Here's the drawing with two shaded views (mm, measured from the low corner). I have some questions. A direction names the side the tool comes from. Coordinates: 2 decimals unless noted, no trailing zeros. Write each loop counter-clockwise with the first axis right and the second up, starting at its lowest first coordinate (ties: lowest second). Pieces come first, ordered by that corner, then holes.
Item 1: If I drill on probe 1 along X at (y, z) = (16, 4.75); probe 2 along Y at (x, z) = (37, 3.05); probe 3 along Y at (x, z) = (15, 3.75), over which ranges is the centre line in solid material (lowest first)?
Item 2: Thinking about a two-plate mould opening in X: for the marked faces 5, 6 and 7, which applies, +X half, -X half, draft (parallel to the pull), parting line (faces both ways), or undercut?
Item 3: Which directions (+Z, -Z, +X, -X, +Y, -Y) give clear straight access to the entire face, cutting with the end or side of a thin tool? Please do the marked faces 1, 2, 3 and 4.
Item 4: I want a section at D-D on y = 1.5. Please give me the cut outline in (x, z), then the cut area to 3 significant figures.
Item 5: I want a section at A-A on z = 1.35. Please give me the cut outline in (x, y).
Item 6: I want a section at C-C on x = 16.5. Please give me the cut outline in (y, z).
Item 7: I want a section at B-B on y = 16.75. Please give me the cut outline in (x, z), then the cut area to 3 significant figures.
Item 8: For P1, Ø5, axis at x = 27.5, y = 18, coming from the -Z side; P2, Ø3, axis at y = 17.5, z = 3.5, coming from the -X side; P3, Ø3, axis at y = 19.5, z = 4, coming from the +X side; P4, Ø1.5, axis at y = 5, z = 2.5, coming from the +X side, each with a flat end and sliding along its axis, tell me the tip position at first contact or that it passes through.
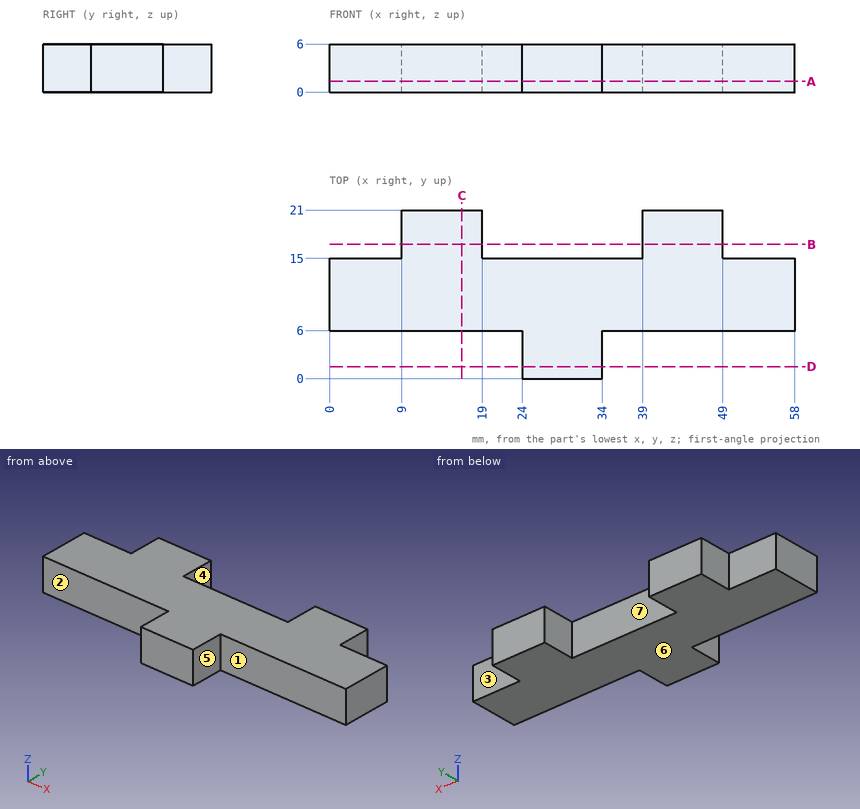
Response values:
1. probe 1: x = 9 to 19, 39 to 49
1. probe 2: y = 6 to 15
1. probe 3: y = 6 to 21
2. face 5: +X half
2. face 6: draft
2. face 7: undercut
3. face 1: +Z, -Z, +X, -Y
3. face 2: +Z, -Z, -X, -Y
3. face 3: +Z, -Z, +X, +Y
3. face 4: +Z, -Z, +Y
4. outline: (24, 0) - (34, 0) - (34, 6) - (24, 6) - close
4. area: 60.0 mm2
5. outline: (0, 6) - (24, 6) - (24, 0) - (34, 0) - (34, 6) - (58, 6) - (58, 15) - (49, 15) - (49, 21) - (39, 21) - (39, 15) - (19, 15) - (19, 21) - (9, 21) - (9, 15) - (0, 15) - close
6. outline: (6, 0) - (21, 0) - (21, 6) - (6, 6) - close
7. outline: (9, 0) - (19, 0) - (19, 6) - (9, 6) - close; (39, 0) - (49, 0) - (49, 6) - (39, 6) - close
7. area: 120 mm2
8. P1: passes through
8. P2: stops at x = 9
8. P3: stops at x = 49
8. P4: stops at x = 34
